Model file for the job. Use its own axes, mm. Face numbers are marked on the shaded views. Coordinates: 2 decimals unless noted, no trailing zeros. Order: outer loops, then holes, each group sorted by start corner. A loop starts at its lowest first (then second) coordinate and runs counter-clockwise, first axis right, second up. Notation, with made-up numbers: (89, 16.5) -> (95, 16.5) arc R16 ccw to (95, 36.5) -> close; hole circle Ø5 at (29.25, 28.25). An arc over 180 degrees is marked (long way). Write item = value, one per line. Start each with the question number.
Q1. Cut at D-D, the plane x = 22. List the corners of the cut face in (y, z).
Q2. Cut at C-C, the plane z = -29. List the corners of the cut face in (x, y).
Q3. Cut at A-A, the plane x = 35. List the corners of the cut face in (y, z).
Q4. Cut at B-B, the plane z = 0. List the corners of the cut face in (x, y).
Q5. Flat gauge pins, fed straight in: pin 1 (4.5 mm diameter, centred on x = 29, z = -53, fed in from -Y); pin 2 (1.5 mm diameter, centred on y = 2, z = -27, fed in from -X); pin 3 (7.5 mm diameter, centred on x = 41.89, z = -78.79, fed in from +Y); pin 4 (1.5 mm diameter, centred on x = 3.5, y = 2, fed in from -Z). Where does each tip first touch, or does it go through?
Q6. Wall check: line 1 (Z direction, x = 39, y = 2.25); line 2 (Z direction, x = 43.5, y = -1.75); line 3 (X direction, y = -1.5, z = -78). Give the ranges that are in metal, low to high. Write a range as from..to.
Q7. Mould opens along Z. For the marked faces 1 and 2 say: +Z half, -Z half, draft (parallel to the pull), parting line (faces both ways), or undercut.
from build123d import *

# Parameters (mm, degrees)
SKETCH1_R                = 1.75
BOSS_EXTRUDE1_DEPTH      = 3
BOSS_EXTRUDE2_DEPTH      = 3
SKETCH3_R                = 4.5
SKETCH3_R_2              = 3.25
BOSS_EXTRUDE3_DEPTH      = 6.2
SKETCH4_R                = 3.25
CUT_EXTRUDE1_DEPTH       = 3
SKETCH5_R                = 7.5
BOSS_EXTRUDE4_DEPTH      = 2
BOSS_EXTRUDE4_DEPTH_BACK = 3
SKETCH6_R                = 4.5
CUT_EXTRUDE2_DEPTH       = 6


with BuildPart() as part:
    # Sketch1 → Boss-Extrude1 (new body)
    with BuildSketch(Plane(origin=(0, 0, 0), x_dir=(1, 0, 0), z_dir=(0, 1, 0))):
        with BuildLine():
            Line((0, -4.5), (10, -4.5))
            ThreePointArc((10, -4.5), (14.5, 0), (10, 4.5))
            Line((10, 4.5), (0, 4.5))
            ThreePointArc((0, 4.5), (-4.5, 0), (0, -4.5))
        make_face()
        Circle(SKETCH1_R, mode=Mode.SUBTRACT)
    extrude(amount=BOSS_EXTRUDE1_DEPTH)

    # Sketch2 → Boss-Extrude2 (add)
    with BuildSketch(Plane(origin=(0, 3, 0), x_dir=(1, 0, 0), z_dir=(0, 1, 0))):
        with BuildLine():
            Line((10, 0), (11.688465713, 4.171220869))
            ThreePointArc((11.688465713, 4.171220869), (10.860088975, 4.41704052), (10, 4.5))
            Line((10, 4.5), (6.96685822, 4.5))
            ThreePointArc((6.96685822, 4.5), (8.346615874, -1.181489024), (14.171220869, -1.688465713))
            Line((14.171220869, -1.688465713), (10, 0))
        make_face()
        with BuildLine():
            ThreePointArc((46.064462111, 77.10126181), (43.648814249, 74.646303405), (40.204775529, 74.618506654))
            Line((40.204775529, 74.618506654), (11.688465713, 4.171220869))
            ThreePointArc((11.688465713, 4.171220869), (14.143424118, 1.755573007), (14.171220869, -1.688465713))
            Line((14.171220869, -1.688465713), (46.064462111, 77.10126181))
        make_face()
        with BuildLine():
            ThreePointArc((14.171220869, -1.688465713), (14.143424118, 1.755573007), (11.688465713, 4.171220869))
            Line((11.688465713, 4.171220869), (10, 0))
            Line((10, 0), (14.171220869, -1.688465713))
        make_face()
        with BuildLine():
            Line((11.688465713, 4.171220869), (40.204775529, 74.618506654))
            ThreePointArc((40.204775529, 74.618506654), (37.749817124, 77.034154516), (37.722020373, 80.478193235))
            Line((37.722020373, 80.478193235), (6.96685822, 4.5))
            Line((6.96685822, 4.5), (10, 4.5))
            ThreePointArc((10, 4.5), (10.860088975, 4.41704052), (11.688465713, 4.171220869))
        make_face()
        with BuildLine():
            Line((37.722020373, 80.478193235), (41.893241242, 78.789727523))
            Line((41.893241242, 78.789727523), (46.064462111, 77.10126181))
            ThreePointArc((46.064462111, 77.10126181), (46.310281762, 77.929638548), (46.393241242, 78.789727523))
            ThreePointArc((46.393241242, 78.789727523), (42.753330217, 83.206768043), (37.722020373, 80.478193235))
        make_face()
        with BuildLine():
            Line((46.064462111, 77.10126181), (41.893241242, 78.789727523))
            Line((41.893241242, 78.789727523), (40.204775529, 74.618506654))
            ThreePointArc((40.204775529, 74.618506654), (43.648814249, 74.646303405), (46.064462111, 77.10126181))
        make_face()
        with BuildLine():
            Line((40.204775529, 74.618506654), (41.893241242, 78.789727523))
            Line((41.893241242, 78.789727523), (37.722020373, 80.478193235))
            ThreePointArc((37.722020373, 80.478193235), (37.749817124, 77.034154516), (40.204775529, 74.618506654))
        make_face()
    extrude(amount=-BOSS_EXTRUDE2_DEPTH)

    # Sketch3 → Boss-Extrude3 (add)
    with BuildSketch(Plane(origin=(0, 3, 0), x_dir=(1, 0, 0), z_dir=(0, 1, 0))):
        with Locations((41.893241242, 78.789727523)):
            Circle(SKETCH3_R)
        with Locations((41.893241242, 78.789727523)):
            Circle(SKETCH3_R_2, mode=Mode.SUBTRACT)
    extrude(amount=-BOSS_EXTRUDE3_DEPTH)

    # Sketch4 → Cut-Extrude1 (cut)
    with BuildSketch(Plane(origin=(0, 3, 0), x_dir=(1, 0, 0), z_dir=(0, 1, 0))):
        with Locations((41.893241242, 78.789727523)):
            Circle(SKETCH4_R)
    extrude(amount=-CUT_EXTRUDE1_DEPTH, mode=Mode.SUBTRACT)

    # Sketch5 → Boss-Extrude4 (add, two sides)
    with BuildSketch(Plane.XZ) as boss_extrude4_sk:
        with Locations((32.137661568, -54.68934028)):
            Circle(SKETCH5_R)
    extrude(amount=BOSS_EXTRUDE4_DEPTH)
    extrude(boss_extrude4_sk.sketch, amount=-BOSS_EXTRUDE4_DEPTH_BACK)

    # Sketch6 → Cut-Extrude2 (cut, through all)
    with BuildSketch(Plane.XZ.offset(2)):
        with Locations((32.137661568, -54.68934028)):
            Circle(SKETCH6_R)
    extrude(amount=-CUT_EXTRUDE2_DEPTH, mode=Mode.SUBTRACT)


solid = part.part
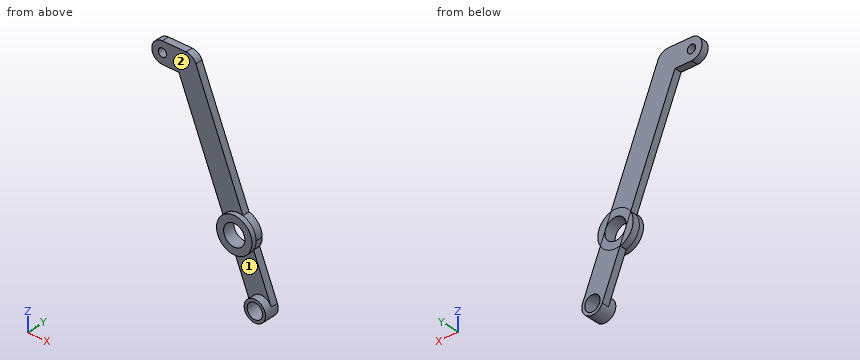
Here are the results:
q1.outline = (0, -41.64) -> (3, -41.64) -> (3, -17.65) -> (0, -17.65) -> close
q2.outline = (16.88, 0) -> (26.59, 0) -> (26.59, 3) -> (16.88, 3) -> close
q3.outline = (-2, -61.62) -> (0, -61.62) -> (0, -73.75) -> (3, -73.75) -> (3, -58.16) -> (-2, -58.16) -> close; (-2, -51.22) -> (3, -51.22) -> (3, -47.76) -> (-2, -47.76) -> close
q4.outline = (-4.5, 0) -> (-1.75, 0) -> (-1.75, 3) -> (-4.5, 3) -> close; (1.75, 0) -> (14.85, 0) -> (14.85, 3) -> (1.75, 3) -> close
q5.pin_1 = -2
q5.pin_2 = 15.77
q5.pin_3 = 3
q5.pin_4 = -4.5
q6.line_1 = -82.24..-80.27, -77.31..-59.65, -57.72..-51.66
q6.line_2 = -82.99..-81.61, -75.96..-74.59
q6.line_3 = 37.46..38.74, 45.05..46.32
q7.face_1 = undercut
q7.face_2 = draft
